from build123d import *

# Parameters (mm, degrees)
BOSS_EXTRU_1_DEPTH         = 6
ESQUISSE2_R                = 9
ESQUISSE2_R_2              = 7.75
ESQUISSE2_R_3              = 3.25
ENL_V_MAT_EXTRU_1_DEPTH    = 191.138226036
ESQUISSE3_W                = 45
ESQUISSE3_H                = 30
ENL_V_MAT_EXTRU_2_DEPTH    = 191.138226036
BOSS_EXTRU_2_DEPTH         = 30
BOSS_EXTRU_3_DEPTH         = 10
ESQUISSE8_R                = 4
ENL_V_MAT_EXTRU_3_DEPTH    = 194.423227664
ENL_V_MAT_EXTRU_4_REACH    = 194.397
ESQUISSE9_R                = 1.35
R_P_TITION_LIN_AIRE1_COUNT = 3
R_P_TITION_LIN_AIRE1_PITCH = 20
ESQUISSE10_R               = 3
ENL_V_MAT_EXTRU_5_DEPTH    = 10
ESQUISSE11_W               = 63
ESQUISSE11_H               = 10
ENL_V_MAT_EXTRU_6_DEPTH    = 5
ESQUISSE12_W               = 10
ESQUISSE12_H               = 87
ENL_V_MAT_EXTRU_7_DEPTH    = 5


with BuildPart() as part:
    # Esquisse1 → Boss.-Extru.1 (new body)
    with BuildSketch(Plane.XY):
        Polygon((0, 0), (63, 0), (154.15, 91.15), (154.15, 111.15), (0, 111.15), align=None)
    extrude(amount=BOSS_EXTRU_1_DEPTH)

    # Esquisse2 → Enlèv. mat.-Extru.1 (cut, through all)
    with BuildSketch(Plane.XY.offset(6)):
        with Locations((49.149999599, 81.15)):
            Circle(ESQUISSE2_R)
        with Locations((74.15, 81.15)):
            Circle(ESQUISSE2_R)
        with Locations((99.15, 81.15)):
            Circle(ESQUISSE2_R)
        with Locations((24.149999599, 81.15)):
            Circle(ESQUISSE2_R)
        with Locations((60, 56)):
            Circle(ESQUISSE2_R_2)
        with Locations((30, 60)):
            Circle(ESQUISSE2_R_3)
        with Locations((15, 60)):
            Circle(ESQUISSE2_R_3)
        Polygon((66.188059223, 39.957611845), (73.966233816, 32.179437252), (90.936796564, 49.15), (83.158621971, 56.928174593), align=None)
    extrude(amount=-ENL_V_MAT_EXTRU_1_DEPTH, mode=Mode.SUBTRACT)

    # Esquisse3 → Enlèv. mat.-Extru.2 (cut, through all)
    with BuildSketch(Plane.XY.offset(6)):
        with Locations((22.5, 30)):
            Rectangle(ESQUISSE3_W, ESQUISSE3_H)
    extrude(amount=-ENL_V_MAT_EXTRU_2_DEPTH, mode=Mode.SUBTRACT)

    # Esquisse6 → Boss.-Extru.2 (add)
    with BuildSketch(Plane(origin=(0, 0, 0), x_dir=(-1, 0, 0), z_dir=(0, 0, -1))):
        Polygon((-154.15, 91.15), (-142.836291501, 91.15), (-59.686291501, 8), (0, 8), (0, 0), (-63, 0), align=None)
    extrude(amount=BOSS_EXTRU_2_DEPTH)

    # Esquisse7 → Boss.-Extru.3 (add)
    with BuildSketch(Plane(origin=(0, 0, 0), x_dir=(-1, 0, 0), z_dir=(0, 0, -1))):
        Polygon((-10, 55), (-45, 55), (-45, 45), (0, 45), (0, 111.15), (-134.15, 111.15), (-134.15, 91.15), (-142.836291501, 91.15), (-128.15, 76.463708499), (-128.15, 105.15), (-10, 105.15), align=None)
    extrude(amount=BOSS_EXTRU_3_DEPTH)

    # Esquisse8 → Enlèv. mat.-Extru.3 (cut, through all)
    with BuildSketch(Plane.XY.offset(6)):
        with Locations((144.15, 101.15)):
            Circle(ESQUISSE8_R)
    extrude(amount=-ENL_V_MAT_EXTRU_3_DEPTH, mode=Mode.SUBTRACT)

    # Esquisse9 → Enlèv. mat.-Extru.4 (cut, up to next)
    with BuildSketch(Plane.ZY, mode=Mode.PRIVATE) as enl_v_mat_extru_4_sk1:
        with Locations((-5, 101.15)):
            Circle(ESQUISSE9_R)
    enl_v_mat_extru_4_tool1 = extrude(enl_v_mat_extru_4_sk1.sketch, amount=-ENL_V_MAT_EXTRU_4_REACH, mode=Mode.PRIVATE) & part.part
    enl_v_mat_extru_4 = enl_v_mat_extru_4_tool1.solids().sort_by_distance((0, 101.15, -5))[0]
    add(enl_v_mat_extru_4, mode=Mode.SUBTRACT)

    # Répétition linéaire1: Enlèv. mat.-Extru.4 ×3
    with Locations(*[(0, -i * R_P_TITION_LIN_AIRE1_PITCH, 0) for i in range(1, R_P_TITION_LIN_AIRE1_COUNT)]):
        add(enl_v_mat_extru_4, mode=Mode.SUBTRACT)

    # Esquisse10 → Enlèv. mat.-Extru.5 (cut)
    with BuildSketch(Plane.ZY):
        with Locations((0, 91.15)):
            Circle(ESQUISSE10_R)
        with Locations((0, 71.15)):
            Circle(ESQUISSE10_R)
        with Locations((0, 51.15)):
            Circle(ESQUISSE10_R)
        with Locations((-14, 4)):
            Circle(ESQUISSE10_R)
        with Locations((0, 4)):
            Circle(ESQUISSE10_R)
    extrude(amount=-ENL_V_MAT_EXTRU_5_DEPTH, mode=Mode.SUBTRACT)

    # Esquisse11 → Enlèv. mat.-Extru.6 (cut)
    with BuildSketch(Plane.XZ):
        with Locations((31.5, -25)):
            Rectangle(ESQUISSE11_W, ESQUISSE11_H)
    extrude(amount=-ENL_V_MAT_EXTRU_6_DEPTH, mode=Mode.SUBTRACT)

    # Esquisse12 → Enlèv. mat.-Extru.7 (cut)
    with BuildSketch(Plane(origin=(31.5, -31.5, 0), x_dir=(0, 0, -1), z_dir=(0.7071067811865489, -0.7071067811865462, 0))):
        with Locations((25, 109.00051032)):
            Rectangle(ESQUISSE12_W, ESQUISSE12_H)
    extrude(amount=-ENL_V_MAT_EXTRU_7_DEPTH, mode=Mode.SUBTRACT)


solid = part.part
CAD build for the part. Positions are in the model's coordinates, mm. A direction names the side the tool comes from. Round coordinates to 2 decimals unless told otherwise and drop trailing zeros. Order: outer loops, then holes, each group sorted by start corner. A loop starts at its lowest first (then second) coordinate and runs counter-clockwise, first axis right, second up. Notation, with made-up numbers: (88, 52.5) -> (137, 52.5) arc R20 ccw to (137, 77.5) -> close; hole circle Ø11 at (-10, -12.75). An arc over 180 degrees is marked (long way). Write each question's results on one line, items separated by ' | '.
1. Pull direction X, two halves, no side cores. Call faces 1 (the face through (22, 15, 3)), 2 (the face through (70, 105.15, -5)), 3 (the face through (63, 2, -25)): pulls with the +X half, pulls with the -X half, needs draft (parallel to the pull), parting line crosses it, or undercut.
Findings below:
face 1: needs draft | face 2: undercut | face 3: pulls with the -X half
2. Cut at C-C (z = -8). Give the cut face in (x, y).
Findings below:
outline: (0, 0) -> (63, 0) -> (154.15, 91.15) -> (134.15, 91.15) -> (134.15, 111.15) -> (0, 111.15) -> (0, 45) -> (45, 45) -> (45, 55) -> (10, 55) -> (10, 105.15) -> (128.15, 105.15) -> (128.15, 76.46) -> (59.69, 8) -> (0, 8) -> close
3. Cut at B-B (x = 99.15). Give the cut face in (y, z).
Findings below:
outline: (36.15, -20) -> (43.22, -20) -> (43.22, -30) -> (47.46, -30) -> (47.46, 0) -> (72.15, 0) -> (72.15, 6) -> (36.15, 6) -> close; (90.15, 0) -> (105.15, 0) -> (105.15, -10) -> (111.15, -10) -> (111.15, 6) -> (90.15, 6) -> close
4. 3-axis set-ups, long thin cutter, end or side, ignore diameter. For faces 4 (the face through (76.07, 16.56, -24.93)), 5 (the face through (140, 101, 0)), 6 (the face through (4.93, 94.124, -0.391)), 7 (the face through (137.59, 78.08, -24.93)), 8 (the face through (70.023, 36.123, 3.042)): which of +Z, -Z, +X, -X, +Y, -Y reach the whole face in a straight line?
Findings below:
face 4: -Z, +X | face 5: -Z, +X, +Y | face 6: -X | face 7: -Z, -Y | face 8: +Z, -Z
5. Flat gauge pins, fed straight in: P1, Ø4, axis at y = 34.5, z = -24, coming from the +X side; P2, Ø10, axis at y = 91.5, z = -2.5, coming from the -X side; P3, Ø5, axis at y = 21.5, z = -9, coming from the -X side; P4, Ø3.5, axis at y = 51.15, z = 0, coming from the -X side. Where does each tip first touch, or does it go through?
Findings below:
P1: stops at x = 92.43 | P2: stops at x = 0 | P3: stops at x = 70.69 | P4: stops at x = 10
6. Cut at A-A (y = 43). Give the cut face in (x, z), plus the area to 3 significant figures.
Findings below:
outline: (45, 0) -> (69.23, 0) -> (69.23, 6) -> (45, 6) -> close; (84.79, 0) -> (94.69, 0) -> (94.69, -30) -> (98.93, -30) -> (98.93, -20) -> (106, -20) -> (106, 6) -> (84.79, 6) -> close | area: 541 mm²
7. Wall check: line 1 along Y through (x, z) = (36, -7.5); line 2 along X through (y, z) = (81, 3); line 3 along Z through (x, y) = (59.5, 79). Give the ranges that are in metal, low to high. Write a range as [from, to].
Findings below:
line 1: y = [0, 8], [45, 55], [105.15, 111.15] | line 2: x = [0, 15.15], [33.15, 40.15], [58.15, 65.15], [83.15, 90.15], [108.15, 144] | line 3: z = [0, 6]
8. Cut at D-D (x = 123). Give the cut face in (y, z), plus the area to 3 significant figures.
Findings below:
outline: (60, -20) -> (67.07, -20) -> (67.07, -30) -> (71.31, -30) -> (71.31, 0) -> (105.15, 0) -> (105.15, -10) -> (111.15, -10) -> (111.15, 6) -> (60, 6) -> close | area: 636 mm²
